Geometry check sheet. Reference: the model listing, model coordinates, mm. A direction names the side the tool comes from. Coordinates: 2 decimals unless noted, no trailing zeros. Write each loop counter-clockwise with the first axis right and the second up, starting at its lowest first coordinate (ties: lowest second). Pieces come first, ordered by that corner, then holes. Notation, with made-up numbers: (77.5, 82) -> (136.5, 82) arc R14 cw to (136.5, 104) -> close; hole circle Ø10 at (24.25, 25). An arc over 180 degrees is marked (long way). One line per question, with ' | ' between items.
```python
from build123d import *

# Parameters (mm, degrees)
SKETCH1_R           = 82.5
SKETCH1_R_2         = 72.5
BOSS_EXTRUDE1_DEPTH = 3
SKETCH2_R           = 5
BOSS_EXTRUDE2_DEPTH = 150


with BuildPart() as part:
    # Sketch1 → Boss-Extrude1 (new body)
    with BuildSketch(Plane(origin=(0, 0, 0), x_dir=(1, 0, 0), z_dir=(0, 1, 0))):
        with Locations(Location((0, 0, 0), (0, 0, 270))):
            Circle(SKETCH1_R)
        with Locations(Location((0, 0, 0), (0, 0, 270))):
            Circle(SKETCH1_R_2, mode=Mode.SUBTRACT)
    extrude(amount=BOSS_EXTRUDE1_DEPTH)

    # Sketch2 → Boss-Extrude2 (add)
    with BuildSketch(Plane(origin=(0, 0, 0), x_dir=(1, 0, 0), z_dir=(0, 1, 0))):
        with Locations(Location((-77.5, 0, 0), (0, 0, 270))):
            Circle(SKETCH2_R)
        with Locations(Location((0, -77.5, 0), (0, 0, 270))):
            Circle(SKETCH2_R)
        with Locations(Location((77.5, 0, 0), (0, 0, 270))):
            Circle(SKETCH2_R)
        with Locations(Location((0, 77.5, 0), (0, 0, 270))):
            Circle(SKETCH2_R)
    extrude(amount=-BOSS_EXTRUDE2_DEPTH)


solid = part.part
```
(1) Cross-section at A-A (z = 12.5). Record the cut outline in (x, y), plus the area to 3 significant figures.
Answers below:
outline: (-81.55, 0) -> (-71.41, 0) -> (-71.41, 3) -> (-81.55, 3) -> close; (71.41, 0) -> (81.55, 0) -> (81.55, 3) -> (71.41, 3) -> close | area: 60.8 mm²
(2) Tool access check on faces 4 (the face through (0, -150, 77)), 5 (the face through (-82.38, -73.95, -1.08)). Record the directions out of +Z, -Z, +X, -X, +Y, -Y that give a thin tool (end or side, any length) a straight path to the whole face; none if there is none.
Answers below:
face 4: +Z, -Z, +X, -X, -Y | face 5: -Y
(3) Cross-section at B-B (x = 43). Record the cut outline in (y, z).
Answers below:
outline: (0, -70.41) -> (3, -70.41) -> (3, -58.37) -> (0, -58.37) -> close; (0, 58.37) -> (3, 58.37) -> (3, 70.41) -> (0, 70.41) -> close
(4) Material ranges on line 1 (Z direction, x = 0, y = 0.6); line 2 (Y direction, x = -73, z = -24), recorded low to high.
Answers below:
line 1: z = -82.5 to -72.5, 72.5 to 82.5 | line 2: y = 0 to 3
(5) Depth check by flat-ended pin: P1, Ø25, axis at x = -57, z = 51.5, coming from the -Y side. Enter the tip coordinate at first touch or a pass-through.
Answers below:
P1: stops at y = 0
(6) Draft check along X on faces 1 (the face through (-1.915, -73.95, 82.119)), 2 (the face through (78, -150, 0)), 3 (the face through (72.62, -73.95, -1.08)). Enter one of: pulls with the +X half, pulls with the -X half, needs draft (parallel to the pull), parting line crosses it, or undercut.
Answers below:
face 1: parting line crosses it | face 2: needs draft | face 3: undercut
(7) Cross-section at D-D (x = -77.5). Record the cut outline in (y, z).
Answers below:
outline: (-150, -5) -> (0, -5) -> (0, -28.28) -> (3, -28.28) -> (3, 28.28) -> (0, 28.28) -> (0, 5) -> (-150, 5) -> close
(8) Cross-section at C-C (y = -62). Record the cut outline in (x, z), plus the area to 3 significant figures.
Answers below:
outline: circle Ø10 at (-77.5, 0); circle Ø10 at (0, -77.5); circle Ø10 at (0, 77.5); circle Ø10 at (77.5, 0) | area: 314 mm²
